Autodesk Inventor part; units mm, degrees
ref_plane "YZ Plane" through (0, 0, 0) normal (1, 0, 0) x (0, 1, 0)
ref_plane "XZ Plane" through (0, 0, 0) normal (0, 1, 0) x (-1, 0, 0)
ref_plane "XY Plane" through (0, 0, 0) normal (0, 0, 1) x (1, 0, 0)
sketch "Sketch1" plane through (0, 0, 0) normal (0, 0, 1) x (1, 0, 0)
  line L0 (92.45, -67.135) -> (-92.45, -67.135) construction
  line L1 (-92.45, -67.135) -> (-92.45, 67.135) construction
  line L2 (-92.45, 67.135) -> (92.45, 67.135) construction
  line L3 (92.45, 67.135) -> (92.45, -67.135) construction
  line L4 (92.45, -67.135) -> (-92.45, 67.135) construction
  line L5 (-92.45, -67.135) -> (92.45, 67.135) construction
  line L6 (77.45, -40.52) -> (-78.55, -40.52) construction
  line L7 (-78.55, -40.52) -> (-78.55, 48.48) construction
  line L8 (-78.55, 48.48) -> (77.45, 48.48) construction
  line L9 (77.45, 48.48) -> (77.45, -40.52) construction
  circle A0 centre (-78.45, 57.48) radius 1.5 construction
  circle A1 centre (-78.45, -57.48) radius 1.5 construction
  line L10 (0, 87.0056) -> (0, -123.2523) construction
  circle A2 centre (78.45, 57.48) radius 1.5 construction
  circle A3 centre (78.45, -57.48) radius 1.5 construction
  line L11 (-78.45, 57.48) -> (78.45, 57.48) construction
  line L12 (-78.45, 57.48) -> (-78.45, 67.135) construction
  line L13 (-78.45, -57.48) -> (-78.45, -67.135) construction
  circle A4 centre (-78.45, 57.48) radius 5
  circle A5 centre (78.45, 57.48) radius 5
  line L14 (-92.45, 0) -> (92.45, 0) construction
  circle A6 centre (-78.45, -57.48) radius 5
  circle A7 centre (78.45, -57.48) radius 5
  line L15 (-81.4051, 53.4467) -> (75.4949, -61.5133)
  line L16 (-75.4949, 61.5133) -> (81.4051, -53.4467)
  line L17 (-75.4949, -61.5133) -> (81.4051, 53.4467)
  line L18 (-81.4051, -53.4467) -> (75.4949, 61.5133)
  point P0 (0, 0)
  point P1 (0, 67.135)
  point P2 (-78.55, 3.98)
  point P3 (0, 57.48)
  dimension "d0" = 184.9
  dimension "d1" = 134.27
  dimension "d2" = 156
  dimension "d3" = 89
  dimension "d4" = 114.96
  dimension "d5" = 3
  dimension "d6" = 156.9
  dimension "d7" = 9
  dimension "d17" = 15
  dimension "d18" = 13.9
  dimension "d19" = 10
extrude "Extrusion3" add sketch "Sketch1" against normal blind 2
sketch "Sketch3" plane through (0, 0, 0) normal (0, 0, 1) x (1, 0, 0)
  circle A0 centre (-78.45, 57.48) radius 5
  line L0 (0, 65.2064) -> (0, -49.8474) construction
  line L1 (-74.1059, 0) -> (81.0801, 0) construction
  arc A1 (-75.4949, 61.5133) -> (-81.4051, 53.4467) centre (-78.45, 57.48) ccw
  circle A2 centre (78.45, 57.48) radius 5
  circle A3 centre (-78.45, -57.48) radius 5
  circle A4 centre (78.45, -57.48) radius 5
  point P0 (0, 0)
extrude "Extrusion4" add sketch "Sketch3" along normal blind 8
sketch "Sketch4" plane through (-78.45, -57.48, 8) normal (0, 0, 1) x (1, 0, 0)
  circle A0 centre (0, 0) radius 1.55
  line L0 (-9.7734, 57.48) -> (187.2333, 57.48) construction
  line L1 (78.45, 128.3827) -> (78.45, -12.8511) construction
  circle A1 centre (156.9, 0) radius 1.55
  circle A2 centre (0, 114.96) radius 1.55
  circle A3 centre (156.9, 114.96) radius 1.55
  circle A4 centre (0, 0) radius 5 construction
  point P0 (78.45, 57.48)
  dimension "d24" = 3.1
extrude "Extrusion5" cut sketch "Sketch4" against normal up to next
sketch "Sketch5" plane through (0, 0, 0) normal (0, 0, 1) x (1, 0, 0)
  line L0 (-29, -24.5) -> (29, -24.5) construction
  line L1 (29, -24.5) -> (29, 24.5) construction
  line L2 (29, 24.5) -> (-29, 24.5) construction
  line L3 (-29, 24.5) -> (-29, -24.5) construction
  line L4 (-29, -24.5) -> (29, 24.5) construction
  line L5 (29, -24.5) -> (-29, 24.5) construction
  circle A0 centre (29, 24.5) radius 1.55
  line L6 (0, 47.6291) -> (0, -68.5673) construction
  line L7 (-80.197, 0) -> (59.821, 0) construction
  circle A1 centre (-29, 24.5) radius 1.55
  line L8 (29, -24.5) -> (-29, -24.5) construction
  circle A2 centre (29, -24.5) radius 1.55
  circle A3 centre (-29, -24.5) radius 1.55
  line L9 (0, 6.1985) -> (-75.4949, 61.5133)
  line L10 (-29.7552, 28) -> (29.7552, 28)
  line L11 (21.5663, 22) -> (-21.5663, 22)
  line L12 (75.4949, 61.5133) -> (0, 6.1985)
  line L13 (-29.7552, -28) -> (29.7552, -28)
  line L14 (21.5663, -22) -> (-21.5663, -22)
  line L15 (-29.7552, -28) -> (-21.5663, -22)
  line L16 (0, -6.1985) -> (-75.4949, -61.5133)
  line L17 (21.5663, -22) -> (29.7552, -28)
  line L18 (75.4949, -61.5133) -> (0, -6.1985)
  point P0 (0, 0)
  dimension "d27" = 58
  dimension "d28" = 49
  dimension "d29" = 3.1
  dimension "d30" = 6
  dimension "d31" = 2.5
extrude "Extrusion6" add sketch "Sketch5" against normal up to surface (2 mm away) contours L9 L10 L12 L11 | L15 L14 L17 L13
extrude "Extrusion7" cut sketch "Sketch5" against normal up to next contours A0 | A1 | A2 | A3
properties part number "LCDv5-backCover"
Here's how the part is built. I have some questions about the finished solid (model axes, mm). A direction names the side the tool comes from. Give positions to 0.01 mm unless a question says otherwise; leave off trailing zeros. Order: outer loops, then holes, each group sorted by start corner. A loop starts at its lowest first (then second) coordinate and runs counter-clockwise, first axis right, second up. Notation, with made-up numbers: (50, 63.5) -> (90, 63.5) arc R18 cw to (90, 90.5) -> close; hole circle Ø11 at (31, -19.5). An arc over 180 degrees is marked (long way). Use CSV: the item, a comma, the result in double quotes. Start each with the question number.
Item 1: On a 3-axis mill with a long thin cutter (end or side, diameter ignored), from which of +Z, -Z, +X, -X, +Y, -Y can I reach the whole of each face in a straight line? I mean faces 1 (the flat face through (10.632, -13.989, -0.986)), 2 (the flat face through (52.3, 44.52, -0.99)), 3 (the flat face through (-77, 59, 8)), 4 (the flat face through (0, -4, -2)), 5 (the cylindrical face through (83.335, 58.545, 3.07)). Say none if no direction works.
Item 2: Suppose I cut it at D-D (x = -57). List the corners of the cut face in (y, z) for me, and give its area (3 significant figures).
Item 3: I'm going to push flat-ended pins straight in: P1, Ø5, axis at x = 19, z = 0, coming from the -Y side; P2, Ø1, axis at x = -3.5, z = -1, coming from the +Y side; P3, Ø3.5, axis at x = 29, y = -24.5, coming from the -Z side; P4, Ø6, axis at x = 52.5, z = 2.5, coming from the +Y side. Where does each tip first touch, or does it pass through?
Item 4: If I drill on probe 1 along Y at (x, z) = (-78.45, 2.5); probe 2 along Y at (x, z) = (-29, -0.65); probe 3 along Z at (x, y) = (39.5, 28), over which ranges is the centre line in solid material (lowest first)? Write a range as [from, to].
Item 5: Thinking about a two-plate mould opening in X: for faces 6 (the flat face through (-52.945, -44.991, -0.986)), 7 (the flat face through (-45.443, 27.097, -0.986)), 8 (the flat face through (44.42, 26.35, -0.99)), 9 (the flat face through (77, -59, 8)), which applies, pulls with the +X half, pulls with the -X half, needs draft (parallel to the pull), parting line crosses it, or undercut?
Item 6: Suppose I cut it at A-A (z = 3.25). List the corners of the cut face in (x, y) for me.
Item 7: Suppose I cut it at C-C (y = 41). List the corners of the cut face in (x, z) for me.
Item 8: Suppose I cut it at B-B (x = -17). List the corners of the cut face in (y, z) for me.
Answer block:
1,face 1,"+Z, -Z"
1,face 2,"+Z, -Z, +Y"
1,face 3,"+Z, +X, -X, +Y, -Y"
1,face 4,"-Z, +X, -X, +Y, -Y"
1,face 5,"+Z"
2,outline,"(-47.96, -2) -> (-35.57, -2) -> (-35.57, 0) -> (-47.96, 0) -> close; (35.57, -2) -> (47.96, -2) -> (47.96, 0) -> (35.57, 0) -> close"
2,area,"49.6 mm^2"
3,P1,"stops at y = -28"
3,P2,"stops at y = 28"
3,P3,"stops at z = -2"
3,P4,"stops at y = 45.88"
4,probe 1,"y = [-62.48, -59.03], [-55.93, -52.48], [52.48, 55.93], [59.03, 62.48]"
4,probe 2,"y = [-28, -26.05], [-22.95, -15.05], [15.05, 22.95], [26.05, 28]"
4,probe 3,"z = [-2, 0]"
5,face 6,"undercut"
5,face 7,"pulls with the -X half"
5,face 8,"pulls with the +X half"
5,face 9,"needs draft"
6,outline,"circle Ø10 at (-78.45, -57.48); circle Ø10 at (-78.45, 57.48); circle Ø10 at (78.45, -57.48); circle Ø10 at (78.45, 57.48); hole circle Ø3.1 at (-78.45, -57.48); hole circle Ø3.1 at (-78.45, 57.48); hole circle Ø3.1 at (78.45, -57.48); hole circle Ø3.1 at (78.45, 57.48)"
7,outline,"(-64.42, -2) -> (-47.5, -2) -> (-47.5, 0) -> (-64.42, 0) -> close; (47.5, -2) -> (64.42, -2) -> (64.42, 0) -> (47.5, 0) -> close"
8,outline,"(-28, -2) -> (-22, -2) -> (-22, 0) -> (-28, 0) -> close; (-18.65, -2) -> (-6.26, -2) -> (-6.26, 0) -> (-18.65, 0) -> close; (6.26, -2) -> (18.65, -2) -> (18.65, 0) -> (6.26, 0) -> close; (22, -2) -> (28, -2) -> (28, 0) -> (22, 0) -> close"
